Part model, mm, in its own coordinate system. A direction names the side the tool comes from. Give positions to 0.01 mm unless a question says otherwise; leave off trailing zeros. Order: outer loops, then holes, each group sorted by start corner. A loop starts at its lowest first (then second) coordinate and runs counter-clockwise, first axis right, second up. Notation, with made-up numbers: M -20,68 L -6,68 A16 ccw -6,82 Z; hole C 81,50.25 d8. An arc over 180 degrees is marked long. Return JSON: item names as keys, results as strings.
from build123d import *

# Parameters (mm, degrees)
SKETCH1_W           = 83
SKETCH1_H           = 15
BOSS_EXTRUDE1_DEPTH = 1.6
SKETCH2_W           = 61
SKETCH2_H           = 15
BOSS_EXTRUDE2_DEPTH = 7.4
SKETCH3_W           = 2
SKETCH3_H           = 13.25
BOSS_EXTRUDE3_DEPTH = 2.25


with BuildPart() as part:
    # Sketch1 → Boss-Extrude1 (new body)
    with BuildSketch(Plane(origin=(0, 0, 0), x_dir=(1, 0, 0), z_dir=(0, 1, 0))):
        Rectangle(SKETCH1_W, SKETCH1_H)
    extrude(amount=BOSS_EXTRUDE1_DEPTH)

    # Sketch2 → Boss-Extrude2 (add)
    with BuildSketch(Plane(origin=(0, 1.6, 0), x_dir=(1, 0, 0), z_dir=(0, 1, 0))):
        Rectangle(SKETCH2_W, SKETCH2_H)
    extrude(amount=BOSS_EXTRUDE2_DEPTH)

    # Sketch3 → Boss-Extrude3 (add)
    with BuildSketch(Plane(origin=(0, 0, 0), x_dir=(-1, 0, 0), z_dir=(0, -1, 0))):
        with Locations((27.5, 0)):
            Rectangle(SKETCH3_W, SKETCH3_H)
    extrude(amount=BOSS_EXTRUDE3_DEPTH)


solid = part.part
Q1. Band-saw the part on B-B (y = 7.25). Give the cut face in (x, z).
Established:
{"outline": "M -30.5,-7.5 L 30.5,-7.5 L 30.5,7.5 L -30.5,7.5 Z"}
Q2. Band-saw the part on A-A (z = 2.5). Give the cut face in (x, y).
Established:
{"outline": "M -41.5,0 L -28.5,0 L -28.5,-2.25 L -26.5,-2.25 L -26.5,0 L 41.5,0 L 41.5,1.6 L 30.5,1.6 L 30.5,9 L -30.5,9 L -30.5,1.6 L -41.5,1.6 Z"}
Q3. Probe line 1 along X through (y, z) = (7, 1.25); line 2 along Y through (x, z) = (-16, -0.25); line 3 along Y through (x, z) = (36.5, 2.75). List the from-to ranges inside material, lowest first.
Established:
{"line 1": "x = -30.5 to 30.5", "line 2": "y = 0 to 9", "line 3": "y = 0 to 1.6"}
Q4. Pin check, flat tips, straight feed: pin 1 (6 mm diameter, centred on y = 7, z = -2, fed in from -X); pin 2 (6 mm diameter, centred on y = 6, z = 1.5, fed in from +X); pin 3 (0.7 mm diameter, centred on y = -1.5, z = 2, fed in from +X); pin 4 (1.1 mm diameter, centred on y = -0.5, z = -3, fed in from -X). Stop position of each tip, or through.
Established:
{"pin 1": "stops at x = -30.5", "pin 2": "stops at x = 30.5", "pin 3": "stops at x = -26.5", "pin 4": "stops at x = -41.5"}
Q5. Band-saw the part on C-C (x = 24.5). Give the cut face in (y, z), then the cut area to 3 significant figures.
Established:
{"outline": "M 0,-7.5 L 9,-7.5 L 9,7.5 L 0,7.5 Z", "area": "135 mm²"}
Q6. 3-axis set-ups, long thin cutter, end or side, ignore diameter. For faces 1 (the flat face through (-28.5, -1, 0)), 2 (the flat face through (-27, -1, 6.625)), 3 (the flat face through (-36, 1.6, 0)), 4 (the flat face through (-27, -1, -6.625)), 5 (the flat face through (-26.5, -1, 0)): which of +Z, -Z, +X, -X, +Y, -Y reach the whole face in a straight line?
Established:
{"face 1": "+Z, -Z, -X, -Y", "face 2": "+Z, +X, -X, -Y", "face 3": "+Z, -Z, -X, +Y", "face 4": "-Z, +X, -X, -Y", "face 5": "+Z, -Z, +X, -Y"}
